Source: CAD feature listing. Evaluate the final solid. Frame: model axes, mm. Round coordinates to 2 decimals unless told otherwise and drop trailing zeros. Order: outer loops, then holes, each group sorted by start corner. A loop starts at its lowest first (then second) coordinate and runs counter-clockwise, first axis right, second up. Notation, with made-up numbers: (76, 23.5) - (108, 23.5) arc R26 cw to (108, 44.5) - close; hole circle Ø4 at (58.25, 30). An arc over 180 degrees is marked (long way). Put each result on its own line as item: value. Start each with the question number.
1) Section A-A on y = 0. Output: boundary loops of the cut face in (x, z).
2) Section C-C on z = -29. Output: boundary loops of the cut face in (x, y).
3) Section D-D on y = -3.5. Output: boundary loops of the cut face in (x, z).
4) Contact query for flat-ended pins moving along their axis: P1, Ø4, axis at x = 29.5, y = -2, coming from the -Z side; P2, Ø1, axis at x = 34, y = -0.5, coming from the -Z side; P3, Ø3, axis at x = 32, y = -1.5, coming from the -Z side; P4, Ø1.5, axis at y = -0.5, z = -17, coming from the -X side. Output: stop coordinate, or through.
5) Line query: probe 1 along Z at (x, y) = (33, -3); probe 2 along Z at (x, y) = (28.5, -1.25); probe 3 along Z at (x, y) = (33.25, 2.5). Output: solid intervals per line, ascending. Write a range as [from, to].
6) Section B-B on x = 30.5. Output: boundary loops of the cut face in (y, z), then the cut area to 3 significant figures.
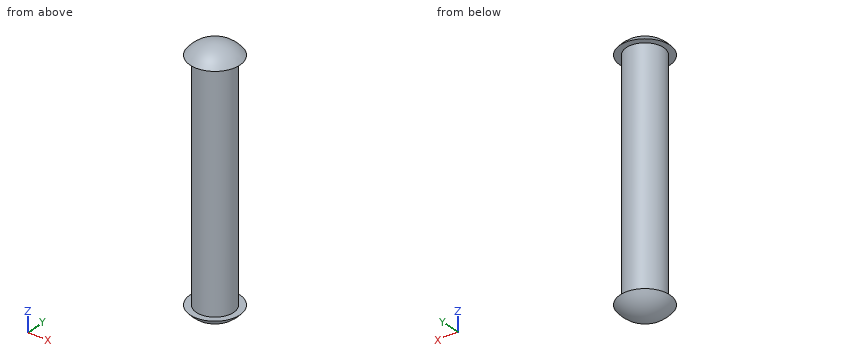
```python
from build123d import *

# Parameters (mm, degrees)
CROQUIS1_R              = 3
SALIENTE_EXTRUIR1_DEPTH = 37


with BuildPart() as part:
    # Croquis1 → Saliente-Extruir1 (new body)
    with BuildSketch(Plane.XY):
        with Locations((31.830127019, 0)):
            Circle(CROQUIS1_R)
    extrude(amount=-SALIENTE_EXTRUIR1_DEPTH)

    # Croquis2 → Revolución1 (revolve)
    with BuildSketch(Plane(origin=(0, 0, 0), x_dir=(1, 0, 0), z_dir=(0, 1, 0))):
        with BuildLine():
            Line((31.830127019, 0), (31.830127019, -2))
            ThreePointArc((31.830127019, -2), (34.066194996, -1.472135955), (35.830127019, 0))
            Line((35.830127019, 0), (31.830127019, 0))
        make_face()
    revoluci_n1 = revolve(axis=Axis((31.830127019, 0, 0), (0, 0, 1)))

    # Simetría1: Revolución1 across plane
    add(revoluci_n1.mirror(Plane.XY.offset(-18.5)))


solid = part.part
```
Answer sheet:
1. outline: (27.83, -37) arc R5 ccw to (35.83, -37) - (34.83, -37) - (34.83, 0) - (35.83, 0) arc R5 ccw to (27.83, 0) - (28.83, 0) - (28.83, -37) - close
2. outline: circle Ø6 at (31.83, 0)
3. outline: (29.89, -37) arc R3.57 ccw to (33.77, -37) - close; (29.89, 0) - (33.77, 0) arc R3.57 ccw to start
4. P1: z = -38.88
4. P2: z = -38.69
4. P3: z = -39
4. P4: x = 28.83
5. probe 1: [-37.83, -37], [0, 0.83]
5. probe 2: [-37.51, -37], [0, 0.51]
5. probe 3: [-38.09, 1.09]
6. outline: (-3.77, -37) arc R4.82 ccw to (3.77, -37) - (2.69, -37) - (2.69, 0) - (3.77, 0) arc R4.82 ccw to (-3.77, 0) - (-2.69, 0) - (-2.69, -37) - close
6. area: 218 mm^2
